from build123d import *

# Parameters (mm, degrees)
F1_DEPTH  = 50
F2_W      = 46
F2_H      = 46
F4_DEPTH  = 1012.001
F5_DEPTH  = 2
F7_DEPTH  = 2
F9_DEPTH  = 2
F11_DEPTH = 2
F12_W     = 10.02
F12_H     = 2.02
F13_DEPTH = 2
F14_W     = 10.02
F14_H     = 2.02
F15_DEPTH = 2


with BuildPart() as f1:
    # F0 (on Front) → F1 (new body)
    with BuildSketch(Plane.XZ):
        Polygon((-36.864701, 862.26987), (-56.864701, 862.26987), (-56.864701, -137.73013), (-36.864701, -137.73013), (-36.864701, -141.73013), (-34.864701, -143.73013), (-28.864701, -143.73013), (-26.864701, -141.73013), (-26.864701, -137.73013), (-6.864701, -137.73013), (-6.864701, 862.26987), (-26.864701, 862.26987), (-26.864701, 866.26987), (-28.864701, 868.26987), (-34.864701, 868.26987), (-36.864701, 866.26987), align=None)
    extrude(amount=F1_DEPTH)

    # F2 (on face) → F4 (cut, through all)
    with BuildSketch(Plane.XY.offset(868.26987)):
        with Locations((-31.864701, -25)):
            Rectangle(F2_W, F2_H)
    extrude(amount=-F4_DEPTH, mode=Mode.SUBTRACT)

    # F3 (on face) → F5 (join)
    with BuildSketch(Plane.YZ.offset(-6.864701)):
        Polygon((-30, 866.26987), (-30, 862.26987), (-20, 862.26987), (-20, 866.26987), (-22, 868.26987), (-28, 868.26987), align=None)
    extrude(amount=-F5_DEPTH)

    # F6 (on face) → F7 (join)
    with BuildSketch(Plane(origin=(-56.864701, 0, 0), x_dir=(0, -1, 0), z_dir=(-1, 0, 0))):
        Polygon((20, 866.26987), (20, 862.26987), (30, 862.26987), (30, 866.26987), (28, 868.26987), (22, 868.26987), align=None)
    extrude(amount=-F7_DEPTH)

    # F8 (on face) → F9 (join)
    with BuildSketch(Plane(origin=(-56.864701, 0, 0), x_dir=(0, -1, 0), z_dir=(-1, 0, 0))):
        Polygon((30, -137.73013), (20, -137.73013), (20, -141.73013), (21.675467, -143.73013), (28.324533, -143.73013), (30, -141.73013), align=None)
    extrude(amount=-F9_DEPTH)

    # F10 (on face) → F11 (join)
    with BuildSketch(Plane.YZ.offset(-6.864701)):
        Polygon((-20, -137.73013), (-30, -137.73013), (-30, -141.73013), (-28, -143.73013), (-22, -143.73013), (-20, -141.73013), align=None)
    extrude(amount=-F11_DEPTH)

    # F12 (on face) → F13 (cut)
    with BuildSketch(Plane.YZ.offset(-6.864701)):
        with Locations((-25, 161.25987)):
            Rectangle(F12_W, F12_H)
        with Locations((-25, 113.27987)):
            Rectangle(F12_W, F12_H)
    extrude(amount=-F13_DEPTH, mode=Mode.SUBTRACT)

    # F14 (on face) → F15 (cut)
    with BuildSketch(Plane(origin=(0, 0, 0), x_dir=(-1, 0, 0), z_dir=(0, 1, 0))):
        with Locations((31.864701, 161.25987)):
            Rectangle(F14_W, F14_H)
        with Locations((31.864701, 113.27987)):
            Rectangle(F14_W, F14_H)
    extrude(amount=-F15_DEPTH, mode=Mode.SUBTRACT)


solid = f1.part
Design review of the part built by this model. Coordinates are the model's own, in mm. A direction names the side the tool comes from. Give positions to 0.01 mm unless a question says otherwise; leave off trailing zeros. Loops run counter-clockwise (first coordinate to the right, second up) from the corner with the lowest first, then second, coordinate; pieces in that order, holes last. Notation, with made-up numbers: (2.25, 89) -> (25.25, 89) arc R15 ccw to (25.25, 96) -> close; hole circle Ø5 at (74.25, -19.75). An arc over 180 degrees is marked (long way). One line per question, with ' | ' between items. Start each with the question number.
(1) For line 1 (X direction, y = -45.5, z = 19.5); line 2 (Y direction, x = -53, z = 265), list the stretches that pass through material, from the lowest coordinate up.
(2) Insertion check: P1, Ø0.6, axis at x = -8, z = 865, coming from the +Y side; P2, Ø16, axis at x = -42.5, y = -8, coming from the -Z side; P3, Ø1, axis at y = -1, z = 865, coming from the +X side. Each pin has a flat end and moves straight along its axis. Give the tip position at first contact, or say it passes through.
(3) For faces 1 (the face through (-13.2, -1.8, -137.73)), 2 (the face through (-55.1, -5.5, -137.73)), 3 (the face through (-55.1, -44.4, -137.73)), list the 3-axis set-ups (+Z, -Z, +X, -X, +Y, -Y) from which the entire face can be reached by the end or side of a thin tool; tool diameter is ignored.
(4) We need section A-A (y = -10). State the section outline as (x, z) points.
(5) We need section B-B (z = 273.5). State the section outline as (x, y) points, and give its area (3 significant figures).
(6) Draft analysis for pull direction Y (two halves, no side actions). For faces 4 (the face through (-54.865, -25, 369)), 5 (the face through (-32, 0, 369)), 6 (the face through (-50.5, -1.8, 862.27)), state which applies: +Y half, -Y half, draft (parallel to the pull), parting line (faces both ways), or undercut.
The answers:
1) line 1: x = -56.86 to -54.86, -8.86 to -6.86 | line 2: y = -50 to -48, -2 to 0
2) P1: stops at y = -20 | P2: stops at z = -137.73 | P3: stops at x = -26.86
3) face 1: -Z, +X, +Y | face 2: -Z, -X, +Y | face 3: -Z, -X, -Y
4) outline: (-56.86, -137.73) -> (-54.86, -137.73) -> (-54.86, 862.27) -> (-56.86, 862.27) -> close; (-8.86, -137.73) -> (-6.86, -137.73) -> (-6.86, 862.27) -> (-8.86, 862.27) -> close
5) outline: (-56.86, -50) -> (-6.86, -50) -> (-6.86, 0) -> (-56.86, 0) -> close; hole (-54.86, -48) -> (-8.86, -48) -> (-8.86, -2) -> (-54.86, -2) -> close | area: 384 mm^2
6) face 4: undercut | face 5: +Y half | face 6: draft
